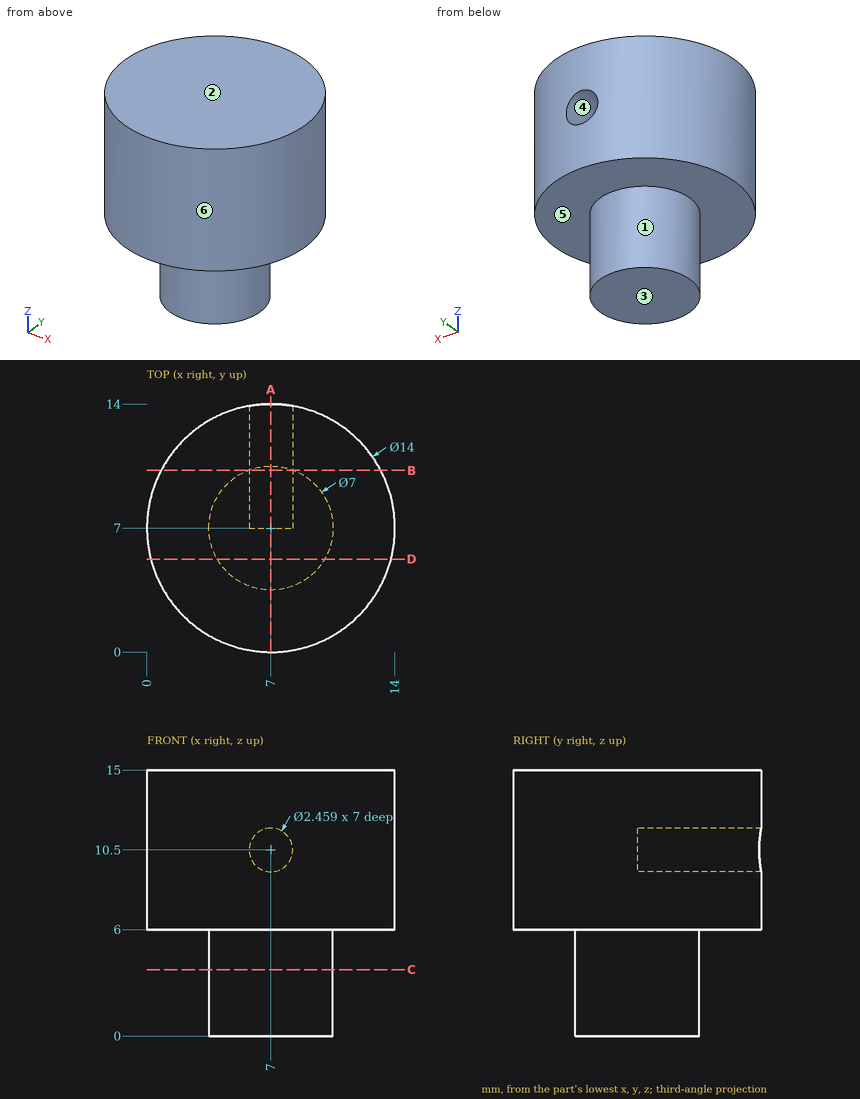
The drawing under review shows one solid part. Ordinate dimensions are in mm from its lowest x, y, z. A direction names the side the tool comes from. Coordinates: 2 decimals unless noted, no trailing zeros. Order: outer loops, then holes, each group sorted by start corner. A loop starts at its lowest first (then second) coordinate and runs counter-clockwise, first axis right, second up. Notation, with made-up numbers: (8, 66) - (20, 66) arc R15 ccw to (20, 90) - close; hole circle Ø7 at (9, 22). An arc over 180 degrees is marked (long way). Put each result on its own line as item: value.
1) Wall thickness on L1, parallel to Z at x = 3, y = 12; L2, parallel to X at y = 10.5, z = 11.25; L3, parallel to X at y = 11, z = 10.5: over which ranges is each line inside the solid? List them lowest first. Write a range as from..to.
Response values:
L1: z = 6..15
L2: x = 0.94..6.03, 7.97..13.06
L3: x = 1.26..5.77, 8.23..12.74
2) The part is to be moulded in two halves that separate along Z. For the marked faces 1, 2, 3 and 4, say which applies: released by +Z, released by -Z, zero draft, split by the parting line, or undercut.
Response values:
face 1: zero draft
face 2: released by +Z
face 3: released by -Z
face 4: undercut
3) Take a section at B-B, the plane y = 10.25. Give the boundary of the cut face in (x, z), and give its area (3 significant figures).
Response values:
outline: (0.8, 6) - (5.7, 6) - (5.7, 0) - (8.3, 0) - (8.3, 6) - (13.2, 6) - (13.2, 15) - (0.8, 15) - close; hole circle Ø2.46 at (7, 10.5)
area: 122 mm²
4) Tool access review of the marked faces 5 and 6: name each direction out of +Z, -Z, +X, -X, +Y, -Y from which nothing blocks a thin tool from reaching the whole face with its end or side.
Response values:
face 5: -Z
face 6: +Z, -Z
5) Insertion check: P1, Ø2, axis at x = 3.5, z = 10.5, coming from the +Y side; P2, Ø1.5, axis at y = 12.5, z = 11, coming from the +X side; P3, Ø2, axis at x = 12.5, z = 12.5, coming from the -Y side. Each pin has a flat end and moves straight along its axis. Give the tip position at first contact, or say it passes through.
Response values:
P1: stops at y = 13.54
P2: stops at x = 12.14
P3: stops at y = 1.64
6) Take a section at D-D, the plane y = 5.25. Give the boundary of the cut face in (x, z), and give its area (3 significant figures).
Response values:
outline: (0.22, 6) - (3.97, 6) - (3.97, 0) - (10.03, 0) - (10.03, 6) - (13.78, 6) - (13.78, 15) - (0.22, 15) - close
area: 158 mm²
7) Take a section at C-C, the plane z = 3.75. Give the boundary of the cut face in (x, y).
Response values:
outline: circle Ø7 at (7, 7)
8) Take a section at A-A, the plane x = 7. Give the boundary of the cut face in (y, z), and give its area (3 significant figures).
Response values:
outline: (0, 6) - (3.5, 6) - (3.5, 0) - (10.5, 0) - (10.5, 6) - (14, 6) - (14, 9.27) - (7, 9.27) - (7, 11.73) - (14, 11.73) - (14, 15) - (0, 15) - close
area: 151 mm²
